For this review, use the dimensioned drawing (mm, ordinates from the lowest corner) and the shaded views. A direction names the side the tool comes from. Coordinates: 2 decimals unless noted, no trailing zeros. Loops run counter-clockwise (first coordinate to the right, second up) from the corner with the lowest first, then second, coordinate; pieces in that order, holes last. Notation, with made-up numbers: M -35,43 L 21,43 A28 ccw 21,76 Z; hole C -31.5,-18 d1. An arc over 180 degrees is marked long. One line per item, written item: value.
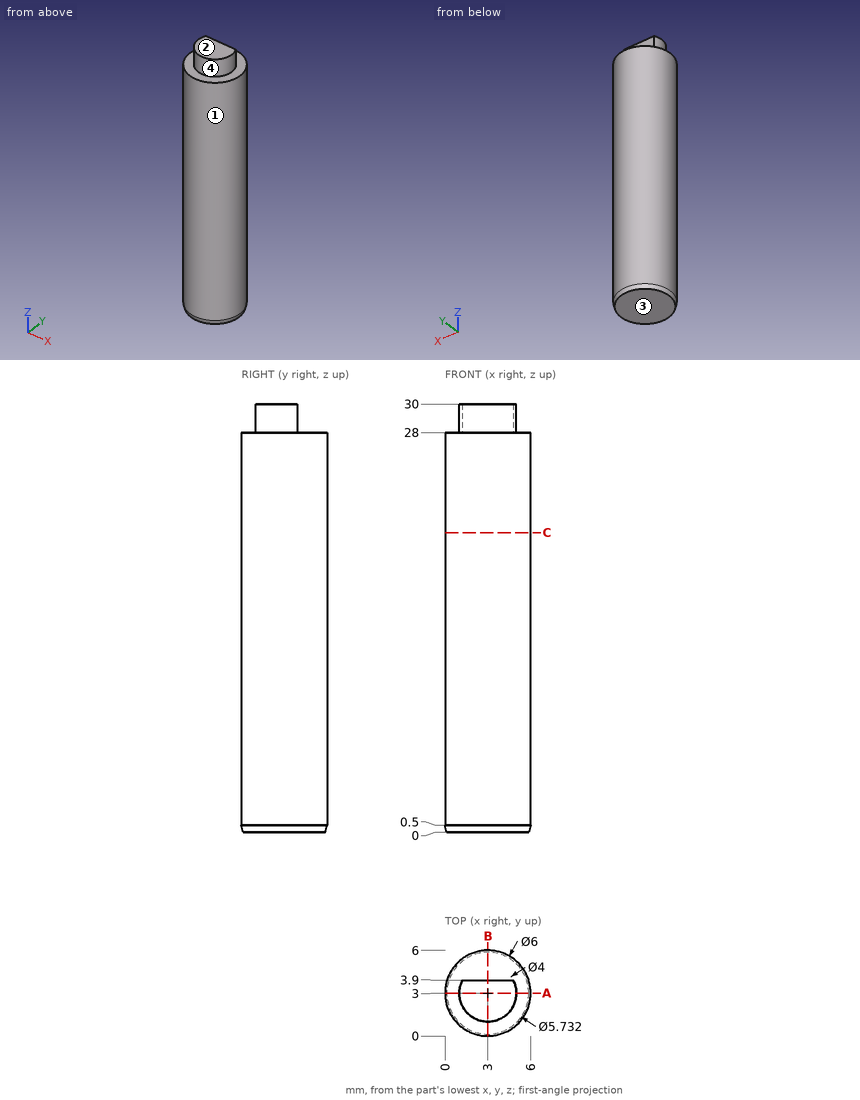
(1) We need section B-B on x = 3. State the section outline as (y, z) points.
Reply:
outline: M 0,0.5 L 0.13,0 L 5.87,0 L 6,0.5 L 6,28 L 3.9,28 L 3.9,30 L 1,30 L 1,28 L 0,28 Z
(2) We need section C-C on z = 21. State the section outline as (x, y) points.
Reply:
outline: C 3,3 d6
(3) To check wall thickness, follow line 1 along Z through (x, y) = (2.15, 4); line 2 along X through (y, z) = (2.8, 13); line 3 along Y through (x, z) = (2.1, 28.5). State the ranges of each line that lie inside material, in increasing order. Write a range as [from, to].
Reply:
line 1: z = [0, 28]
line 2: x = [0.01, 5.99]
line 3: y = [1.21, 3.9]
(4) Tool access review of the marked faces 3 and 4: name each direction out of +Z, -Z, +X, -X, +Y, -Y from which nothing blocks a thin tool from reaching the whole face with its end or side.
Reply:
face 3: -Z, +X, -X, +Y, -Y
face 4: +Z
(5) Mouldability with a two-part tool opening along X and no side actions: class the marked faces 1 and 2 as released by +X, released by -X, zero draft, split by the parting line, or undercut.
Reply:
face 1: split by the parting line
face 2: zero draft
(6) We need section A-A on y = 3. State the section outline as (x, z) points.
Reply:
outline: M 0,0.5 L 0.13,0 L 5.87,0 L 6,0.5 L 6,28 L 5,28 L 5,30 L 1,30 L 1,28 L 0,28 Z
(7) Insertion check: pin 1 (1 mm diameter, centred on x = 2.5, z = 29, fed in from +Y); pin 2 (1 mm diameter, centred on y = 1.5, z = 15.5, fed in from -X). Each pin has a flat end and moves straight along its axis. Give the tip position at first contact, or say it passes through.
Reply:
pin 1: stops at y = 3.9
pin 2: stops at x = 0.17
